Verification items for this drawing (mm, ordinates from the low corner). A direction names the side the tool comes from. Coordinates: 2 decimals unless noted, no trailing zeros. Use CSV: the item, a comma, the result in double quotes.
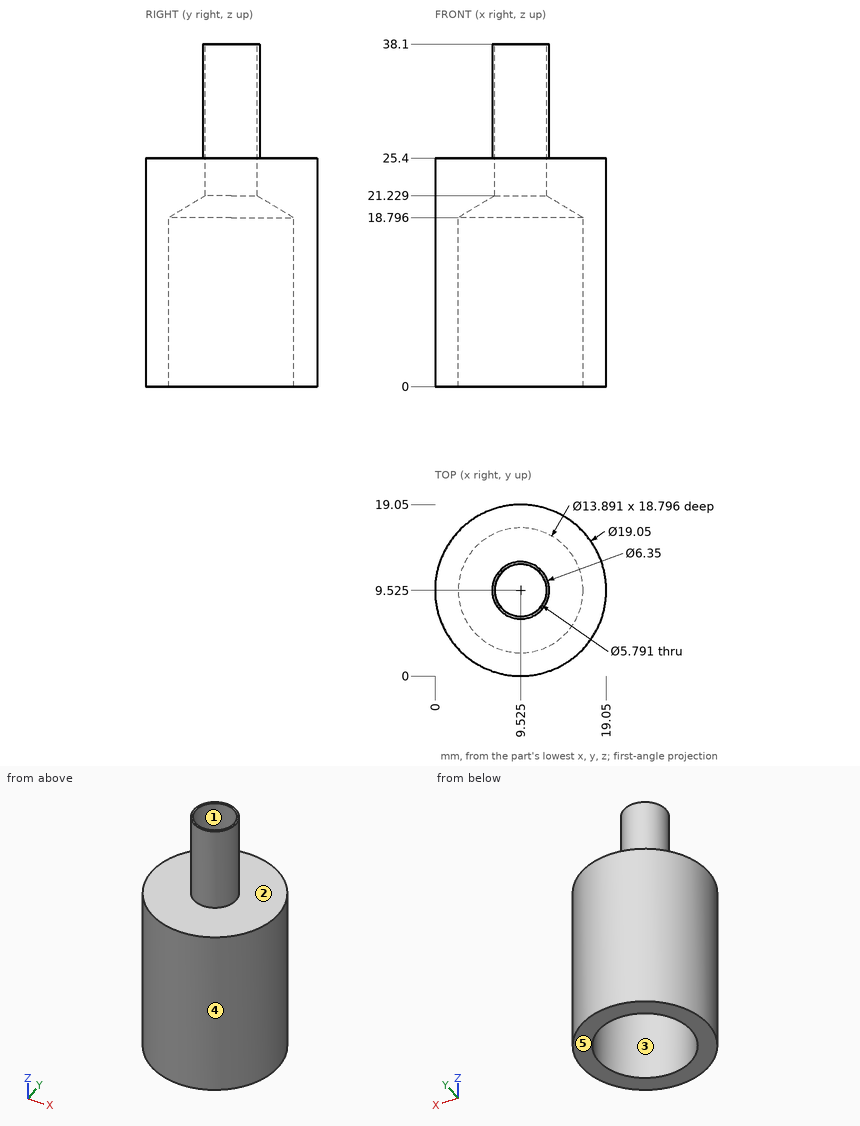
1. Set-up check for the marked faces 1 and 2: record each of +Z, -Z, +X, -X, +Y, -Y from which the full face is reachable in a straight line by a thin tool's end or side.
The answers:
face 1,"+Z, -Z"
face 2,"+Z"
2. Release check for a two-part mould opening along Y. For the marked faces 3, 4 and 5 record: +Y half, -Y half, draft (parallel to the pull), parting line (faces both ways), or undercut.
The answers:
face 3,"undercut"
face 4,"parting line"
face 5,"draft"
3. Gauge pin test, flat ends, axial feed: P1, Ø8, axis at x = 17, y = 12.5, coming from the +Z side; P2, Ø8, axis at y = 16.5, z = 27.5, coming from the +X side (1 decimal); P3, Ø8, axis at x = 10.5, y = 9.5, coming from the -Z side. Record the tip position at first contact, or that the pin passes through.
The answers:
P1,"z = 25.4"
P2,"x = 18.4"
P3,"z = 19.98"
4. Thickness scan on line 1 (Y direction, x = 9.5, z = 35.5); line 2 (Z direction, x = 9.25, y = 3) (1 decimal); line 3 (X direction, y = 10, z = 30.5) (1 decimal). Record the ranges inside material, lowest first. Write a range as [from, to].
The answers:
line 1,"[6.35, 6.63], [12.42, 12.7]"
line 2,"[19, 25.4]"
line 3,"[6.4, 6.7], [12.4, 12.7]"
